```python
from build123d import *

# Parameters (mm, degrees)
EXTRUDE_1_DEPTH       = 244
EXTRUDE_3_DEPTH       = 244
PATTERN_CURVE_1_DEPTH = 244
SKETCH_3_R            = 2.25
CUT_EXTRUDE_1_DEPTH   = 6
SKETCH_4_R            = 1.6
SKETCH_4_R_2          = 1.3
CUT_EXTRUDE_2_DEPTH   = 6


# Read off the part's stored shape, not the designer's step: the pattern curve step
with BuildPart() as part:
    # Sketch 1 → Extrude 1 (new body)
    with BuildSketch(Plane.XY):
        with BuildLine():
            Line((0, 40), (1.528979332, 40))
            ThreePointArc((1.528979332, 40), (2.225614441, 39.717425624), (2.528547087, 39.029399052))
            Line((2.528547087, 39.029399052), (3.5, 6))
            Line((3.5, 6), (118.5, 6))
            Line((118.5, 6), (119.471452913, 39.029399052))
            ThreePointArc((119.471452913, 39.029399052), (119.774385559, 39.717425624), (120.471020668, 40))
            Line((120.471020668, 40), (122, 40))
            Line((122, 40), (122, 0))
            Line((122, 0), (0, 0))
            Line((0, 0), (0, 40))
        make_face()
    extrude(amount=EXTRUDE_1_DEPTH)

    # Sketch 2 → Extrude 3 (add)
    with BuildSketch(Plane.XY.offset(244)):
        with BuildLine():
            Line((10.5, 39.5), (9.25, 6))
            Line((9.25, 6), (12.75, 6))
            Line((12.75, 6), (11.5, 39.5))
            ThreePointArc((11.5, 39.5), (11, 40), (10.5, 39.5))
        make_face()
    extrude(amount=-EXTRUDE_3_DEPTH)

    # Pattern Curve 1 outline → Pattern Curve 1 (add)
    with BuildSketch(Plane.XY):
        with BuildLine():
            ThreePointArc((21.5, 39.5), (21, 40), (20.5, 39.5))
            Line((20.5, 39.5), (19.25, 6))
            Line((19.25, 6), (22.75, 6))
            Line((22.75, 6), (21.5, 39.5))
        make_face()
        with BuildLine():
            Line((110.5, 39.5), (109.25, 6))
            Line((109.25, 6), (112.75, 6))
            Line((112.75, 6), (111.5, 39.5))
            ThreePointArc((111.5, 39.5), (111, 40), (110.5, 39.5))
        make_face()
        with BuildLine():
            Line((100.5, 39.5), (99.25, 6))
            Line((99.25, 6), (102.75, 6))
            Line((102.75, 6), (101.5, 39.5))
            ThreePointArc((101.5, 39.5), (101, 40), (100.5, 39.5))
        make_face()
        with BuildLine():
            Line((90.5, 39.5), (89.25, 6))
            Line((89.25, 6), (92.75, 6))
            Line((92.75, 6), (91.5, 39.5))
            ThreePointArc((91.5, 39.5), (91, 40), (90.5, 39.5))
        make_face()
        with BuildLine():
            Line((80.5, 39.5), (79.25, 6))
            Line((79.25, 6), (82.75, 6))
            Line((82.75, 6), (81.5, 39.5))
            ThreePointArc((81.5, 39.5), (81, 40), (80.5, 39.5))
        make_face()
        with BuildLine():
            Line((70.5, 39.5), (69.25, 6))
            Line((69.25, 6), (72.75, 6))
            Line((72.75, 6), (71.5, 39.5))
            ThreePointArc((71.5, 39.5), (71, 40), (70.5, 39.5))
        make_face()
        with BuildLine():
            Line((60.5, 39.5), (59.25, 6))
            Line((59.25, 6), (62.75, 6))
            Line((62.75, 6), (61.5, 39.5))
            ThreePointArc((61.5, 39.5), (61, 40), (60.5, 39.5))
        make_face()
        with BuildLine():
            Line((50.5, 39.5), (49.25, 6))
            Line((49.25, 6), (52.75, 6))
            Line((52.75, 6), (51.5, 39.5))
            ThreePointArc((51.5, 39.5), (51, 40), (50.5, 39.5))
        make_face()
        with BuildLine():
            Line((40.5, 39.5), (39.25, 6))
            Line((39.25, 6), (42.75, 6))
            Line((42.75, 6), (41.5, 39.5))
            ThreePointArc((41.5, 39.5), (41, 40), (40.5, 39.5))
        make_face()
        with BuildLine():
            Line((30.5, 39.5), (29.25, 6))
            Line((29.25, 6), (32.75, 6))
            Line((32.75, 6), (31.5, 39.5))
            ThreePointArc((31.5, 39.5), (31, 40), (30.5, 39.5))
        make_face()
    extrude(amount=PATTERN_CURVE_1_DEPTH)

    # Sketch 3 → Cut-Extrude 1 (cut)
    with BuildSketch(Plane.XZ):
        with Locations((26, 236)):
            Circle(SKETCH_3_R)
        with Locations((96, 236)):
            Circle(SKETCH_3_R)
        with Locations(Location((96, 8, 0), (0, 0, 180))):
            Circle(SKETCH_3_R)
        with Locations(Location((26, 8, 0), (0, 0, 180))):
            Circle(SKETCH_3_R)
    extrude(amount=-CUT_EXTRUDE_1_DEPTH, mode=Mode.SUBTRACT)

    # Sketch 4 → Cut-Extrude 2 (cut)
    with BuildSketch(Plane(origin=(133.240090243, 0, 310.149074448), x_dir=(-1, 0, 0), z_dir=(0, -1, 0))):
        with Locations(Location((71.240090243, 92.149074448, 0), (0, 0, 180))):
            Circle(SKETCH_4_R)
        with Locations(Location((71.240090243, 227.149074448, 0), (0, 0, 180))):
            Circle(SKETCH_4_R)
        with Locations(Location((31.490090243, 223.549074448, 0), (0, 0, 180))):
            Circle(SKETCH_4_R)
        with Locations(Location((31.490090243, 139.749074448, 0), (0, 0, 180))):
            Circle(SKETCH_4_R)
        with Locations(Location((34.240090243, 100.649074448, 0), (0, 0, 180))):
            Circle(SKETCH_4_R_2)
        with Locations(Location((91.240090243, 285.149074448, 0), (0, 0, 180))):
            Circle(SKETCH_4_R)
        with Locations(Location((91.240090243, 237.149074448, 0), (0, 0, 180))):
            Circle(SKETCH_4_R)
        with Locations(Location((25.240090243, 237.149074448, 0), (0, 0, 180))):
            Circle(SKETCH_4_R)
        with Locations(Location((25.240090243, 285.149074448, 0), (0, 0, 180))):
            Circle(SKETCH_4_R)
    extrude(amount=-CUT_EXTRUDE_2_DEPTH, mode=Mode.SUBTRACT)


solid = part.part
```
For this review, take the finished solid that the model builds, in its own axes (mm). A direction names the side the tool comes from. Round coordinates to 2 decimals unless told otherwise and drop trailing zeros.
(1) Wall thickness on line 1 along Z through (x, y) = (62, 3.55); line 2 along X through (y, z) = (4, 236); line 3 along Z through (x, y) = (96, 4.2): over which ranges is each line inside the solid? List them lowest first.
Returned:
line 1: z = 0 to 81.4, 84.6 to 216.4, 219.6 to 244
line 2: x = 0 to 23.75, 28.25 to 93.75, 98.25 to 122
line 3: z = 0 to 5.75, 10.25 to 233.75, 238.25 to 244
(2) Clearance check with flat-ended pins moving along their axes: P1, Ø5, axis at x = 26, z = 236, coming from the +Y side; P2, Ø10, axis at x = 59.5, z = 107, coming from the -Y side. State where each tip first meets the part, or that it passes through.
Returned:
P1: stops at y = 6
P2: stops at y = 0
(3) We need section A-A (z = 8). State how many separate pieces and enclosed holes the cut face has, plus the area to 3 significant figures.
Returned:
separate pieces: 3
enclosed holes: 0
area: 1,720 mm2
(4) Tool access review of faces 1 (the flat face through (26, 6, 120)), 2 (the cylindrical face through (25.71, 2.96, 238.23)): name each direction out of +Z, -Z, +X, -X, +Y, -Y from which nothing blocks a thin tool from reaching the whole face with its end or side.
Returned:
face 1: +Z, -Z, +Y
face 2: +Y, -Y
